from build123d import *

# Parameters (mm, degrees)
F0_W     = 1700
F0_H     = 1830
F1_DEPTH = 365
F2_W     = 1500
F2_H     = 1630
F3_DEPTH = 630
F4_DEPTH = 25
F5_W     = 200
F5_H     = 85
F6_DEPTH = 1630


with BuildPart() as f1:
    # F0 (on Front) → F1 (new body, symmetric)
    with BuildSketch(Plane.XZ):
        Rectangle(F0_W, F0_H)
    extrude(amount=F1_DEPTH, both=True)

    # F2 (on face) → F3 (cut)
    with BuildSketch(Plane.XZ.offset(365)):
        Rectangle(F2_W, F2_H)
    extrude(amount=-F3_DEPTH, mode=Mode.SUBTRACT)

    # F4 (add): a face of the model
    f4_faces = [f1.faces().sort_by_distance(p)[0] for p in [
        (0, -50, -815),
    ]]
    extrude(f4_faces, amount=F4_DEPTH)

    # F5 (on face) → F6 (join)
    with BuildSketch(Plane.XY.offset(-790)):
        with Locations((0, -322.5)):
            Rectangle(F5_W, F5_H)
    extrude(amount=F6_DEPTH)


solid = f1.part
Build history of the part. All positions in model axes, mm. A direction names the side the tool comes from. Round coordinates to 2 decimals unless told otherwise and drop trailing zeros. Loops run counter-clockwise (first coordinate to the right, second up) from the corner with the lowest first, then second, coordinate; pieces in that order, holes last. Notation, with made-up numbers: (9.25, 74) -> (53.25, 74) arc R23 cw to (53.25, 88) -> close; hole circle Ø8 at (78.25, 12.5). An arc over 180 degrees is marked (long way). Use CSV: the item, a comma, the result in double quotes. Start each with the question number.
Q1. Saw through at D-D on x = -409.5. Give the cut face in (y, z).
Q2. Saw through at A-A on y = -130.5. Give the cut face in (x, z).
Q3. Which spindle directions (+Z, -Z, +X, -X, +Y, -Y) get a long thin tool onto all of the face, cutting with end or side? Do faces 1 (the face through (-1, -280, 1)), 2 (the face through (-12, -5, -915)), 3 (the face through (-100, -323, 1)). Say none if no direction does.
Q4. Drill centre lines: L1, parallel to X at y = -115.5, z = 38; L2, parallel to Z at x = 528, y = -154; L3, parallel to Y at x = 660, z = -205.5. Where is each one in solid material? Low to high.
Q5. Mould opens along Z. For faces 4 (the face through (-10, 265, 24)), 5 (the face through (-12, -5, 915)), 6 (the face through (-4, -365, -72)) say: +Z half, -Z half, draft (parallel to the pull), parting line (faces both ways), or undercut.
Q6. Saw through at B-B on z = 154.5. Give the cut face in (x, y).
Q7. Saw through at C-C on x = -19. Give the cut face in (y, z).
Solutions:
1,outline,"(-365, -915) -> (365, -915) -> (365, 915) -> (-365, 915) -> (-365, 815) -> (265, 815) -> (265, -790) -> (-365, -790) -> close"
2,outline,"(-850, -915) -> (850, -915) -> (850, 915) -> (-850, 915) -> close; hole (-750, -790) -> (750, -790) -> (750, 815) -> (-750, 815) -> close"
3,face 1,"none"
3,face 2,"-Z, +X, -X, +Y, -Y"
3,face 3,"-Y"
4,L1,"x = -850 to -750, 750 to 850"
4,L2,"z = -915 to -790, 815 to 915"
4,L3,"y = 265 to 365"
5,face 4,"undercut"
5,face 5,"+Z half"
5,face 6,"draft"
6,outline,"(-850, -365) -> (-750, -365) -> (-750, 265) -> (750, 265) -> (750, -365) -> (850, -365) -> (850, 365) -> (-850, 365) -> close; (-100, -365) -> (100, -365) -> (100, -280) -> (-100, -280) -> close"
7,outline,"(-365, -915) -> (365, -915) -> (365, 915) -> (-365, 915) -> close; hole (-280, -790) -> (265, -790) -> (265, 815) -> (-280, 815) -> close"
